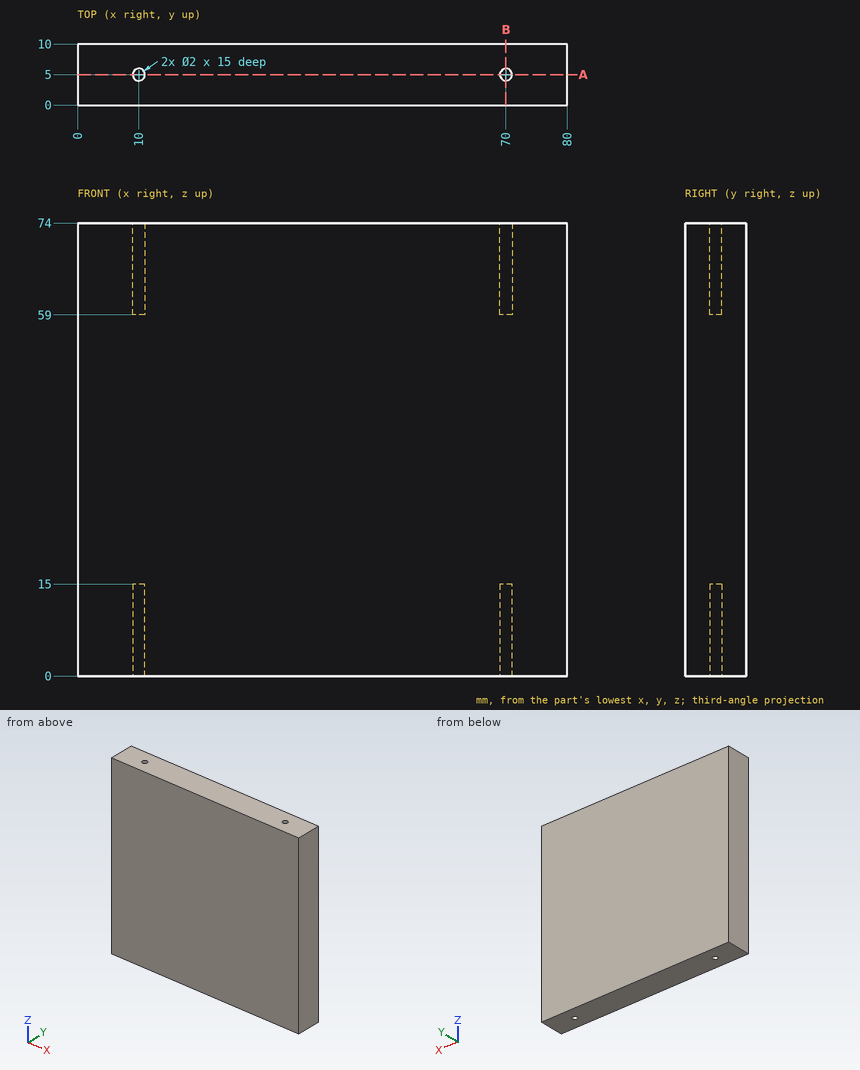
Geometry check sheet. Reference: drawing and pictorial views, mm from the part's lowest x, y, z. Give positions to 0.01 mm unless a question says otherwise; leave off trailing zeros. Write each loop counter-clockwise with the first axis right and the second up, starting at its lowest first coordinate (ties: lowest second). Pieces come first, ordered by that corner, then holes. Notation, with made-up numbers: M 22,-2.5 L 40,-2.5 A27 ccw 40,27.5 Z; hole C -1.75,20.5 d8. An arc over 180 degrees is marked long. Put each result on its own line as item: value. Start each with the question number.
1. Scan line: line 1 along Y through (x, z) = (70, 4.75). Record every from-to range of solid material in increasing order. Write a range as [from, to].
2. Section check A-A (y = 5). Record the cut outline in (x, z), and give its area (3 significant figures).
3. Section check B-B (x = 70). Record the cut outline in (y, z), and give its area (3 significant figures).
4. Go/stop test with flat-tipped pins: pin 1 Ø1.2 at (x, y) = (70, 5) entering from -Z; pin 2 Ø0.6 at (x, y) = (10, 5) entering from +Z. Record where each tip stops, or that it passes through.
Answer list:
1. line 1: [0, 4], [6, 10]
2. outline: M 0,0 L 9,0 L 9,15 L 11,15 L 11,0 L 69,0 L 69,15 L 71,15 L 71,0 L 80,0 L 80,74 L 71,74 L 71,59 L 69,59 L 69,74 L 11,74 L 11,59 L 9,59 L 9,74 L 0,74 Z
2. area: 5,800 mm2
3. outline: M 0,0 L 4,0 L 4,15 L 6,15 L 6,0 L 10,0 L 10,74 L 6,74 L 6,59 L 4,59 L 4,74 L 0,74 Z
3. area: 680 mm2
4. pin 1: z = 15
4. pin 2: z = 59
